from build123d import *

# Parameters (mm, degrees)
SKETCH1_R           = 1.45
BOSS_EXTRUDE1_DEPTH = 8
SKETCH2_R           = 4
SKETCH2_R_2         = 1.45
BOSS_EXTRUDE2_DEPTH = 2
SKETCH4_R           = 4
SKETCH4_R_2         = 2.75
BOSS_EXTRUDE3_DEPTH = 3
CUT_EXTRUDE1_DEPTH  = 3
CUT_EXTRUDE2_REACH  = 73.014
SKETCH6_R           = 1.5
CUT_EXTRUDE3_DEPTH  = 3
BOSS_EXTRUDE8_DEPTH = 5
BOSS_EXTRUDE9_START = -11
BOSS_EXTRUDE9_DEPTH = 4
CUT_EXTRUDE6_DEPTH  = 72.01408311
SKETCH6_7_R         = 1.5
CUT_EXTRUDE7_DEPTH  = 3


with BuildPart() as part:
    # Sketch1 → Boss-Extrude1 (new body)
    with BuildSketch(Plane(origin=(0, 0, 0), x_dir=(1, 0, 0), z_dir=(0, 1, 0))):
        with BuildLine():
            Line((-7.5, 36.5), (-43, 36.5))
            Line((-43, 36.5), (-43, 32.5))
            Line((-43, 32.5), (-17.5, 32.5))
            ThreePointArc((-17.5, 32.5), (-10.428932188, 29.571067812), (-7.5, 22.5))
            Line((-7.5, 22.5), (-7.5, 0))
            ThreePointArc((-7.5, 0), (0, -7.5), (7.5, 0))
            Line((7.5, 0), (7.5, 40))
            ThreePointArc((7.5, 40), (5.303300859, 45.303300859), (0, 47.5))
            Line((0, 47.5), (-19, 47.5))
            Line((-19, 47.5), (-19, 42.5))
            Line((-19, 42.5), (-7.5, 42.5))
            Line((-7.5, 42.5), (-7.5, 36.5))
        make_face()
        with Locations(Location((0, 0, 0), (0, 0, 270))):
            Circle(SKETCH1_R, mode=Mode.SUBTRACT)
        with BuildLine():
            ThreePointArc((-3.822328563, 25.208378945), (-4.975312132, 23.472395947), (-3.280610142, 22.259550844))
            ThreePointArc((-3.280610142, 22.259550844), (-0.06671842, 22.49990123), (3.148542183, 22.278615056))
            ThreePointArc((3.148542183, 22.278615056), (4.95957959, 23.370856111), (3.89359262, 25.197470135))
            ThreePointArc((3.89359262, 25.197470135), (0.03604708, 25.496495157), (-3.822328563, 25.208378945))
        make_face(mode=Mode.SUBTRACT)
    extrude(amount=BOSS_EXTRUDE1_DEPTH)

    # Sketch2 → Boss-Extrude2 (add)
    with BuildSketch(Plane(origin=(0, 8, 0), x_dir=(1, 0, 0), z_dir=(0, 1, 0))):
        with Locations(Location((0, 0, 0), (0, 0, 270))):
            Circle(SKETCH2_R)
        with Locations(Location((0, 0, 0), (0, 0, 270))):
            Circle(SKETCH2_R_2, mode=Mode.SUBTRACT)
    extrude(amount=BOSS_EXTRUDE2_DEPTH)

    # Sketch4 → Boss-Extrude3 (add)
    with BuildSketch(Plane(origin=(0, 10, 0), x_dir=(1, 0, 0), z_dir=(0, 1, 0))):
        with Locations(Location((0, 0, 0), (0, 0, 270))):
            Circle(SKETCH4_R)
        with Locations(Location((0, 0, 0), (0, 0, 270))):
            Circle(SKETCH4_R_2, mode=Mode.SUBTRACT)
    extrude(amount=BOSS_EXTRUDE3_DEPTH)

    # Sketch5 → Cut-Extrude1 (cut)
    with BuildSketch(Plane(origin=(0, 8, 0), x_dir=(1, 0, 0), z_dir=(0, 1, 0))):
        with BuildLine():
            ThreePointArc((-3.901041667, 26.464020366), (-6.220600225, 23.342378475), (-3.098958333, 21.022819917))
            ThreePointArc((-3.098958333, 21.022819917), (0, 21.25), (3.098958333, 21.022819917))
            ThreePointArc((3.098958333, 21.022819917), (6.220600225, 23.342378475), (3.901041667, 26.464020366))
            ThreePointArc((3.901041667, 26.464020366), (0, 26.75), (-3.901041667, 26.464020366))
        make_face()
    extrude(amount=-CUT_EXTRUDE1_DEPTH, mode=Mode.SUBTRACT)

    # Sketch6 → Cut-Extrude2 (cut, up to next)
    with BuildSketch(Plane(origin=(0, 0, -47.5), x_dir=(-1, 0, 0), z_dir=(0, 0, -1)), mode=Mode.PRIVATE) as cut_extrude2_sk1:
        with Locations((35, 4)):
            Circle(SKETCH6_R)
    cut_extrude2_tool1 = extrude(cut_extrude2_sk1.sketch, amount=-CUT_EXTRUDE2_REACH, mode=Mode.PRIVATE) & part.part
    # Sketch6 → Cut-Extrude2 (cut, up to next)
    with BuildSketch(Plane(origin=(0, 0, -47.5), x_dir=(-1, 0, 0), z_dir=(0, 0, -1)), mode=Mode.PRIVATE) as cut_extrude2_sk2:
        with BuildLine():
            ThreePointArc((13.205467269, 9.590021738), (12.125166536, 11.415658703), (10.299529571, 10.33535797))
            ThreePointArc((10.299529571, 10.33535797), (9.639691668, 6.665475813), (9.522099126, 2.938601373))
            ThreePointArc((9.522099126, 2.938601373), (11.083234391, 1.502336535), (12.519499229, 3.0634718))
            ThreePointArc((12.519499229, 3.0634718), (12.623257354, 6.351890424), (13.205467269, 9.590021738))
        make_face()
    cut_extrude2_tool2 = extrude(cut_extrude2_sk2.sketch, amount=-CUT_EXTRUDE2_REACH, mode=Mode.PRIVATE) & part.part
    add(cut_extrude2_tool1.solids().sort_by_distance((-35, 4, -47.5))[0], mode=Mode.SUBTRACT)
    add(cut_extrude2_tool2.solids().sort_by_distance((-11.259305, 6.495248, -47.5))[0], mode=Mode.SUBTRACT)

    # Sketch6<3> → Cut-Extrude3 (cut)
    with BuildSketch(Plane(origin=(0, 0, -47.5), x_dir=(-1, 0, 0), z_dir=(0, 0, -1))):
        with BuildLine():
            ThreePointArc((9.088722197, 10.645914733), (8.396539299, 6.796136392), (8.273182416, 2.886572028))
            ThreePointArc((8.273182416, 2.886572028), (11.135263735, 0.253419825), (13.768415938, 3.115501144))
            ThreePointArc((13.768415938, 3.115501144), (13.866409723, 6.221229844), (14.416274643, 9.279464975))
            ThreePointArc((14.416274643, 9.279464975), (12.435723299, 12.626466077), (9.088722197, 10.645914733))
        make_face()
        with BuildLine():
            ThreePointArc((10.299529571, 10.33535797), (9.639691668, 6.665475813), (9.522099126, 2.938601373))
            ThreePointArc((9.522099126, 2.938601373), (11.083234391, 1.502336535), (12.519499229, 3.0634718))
            ThreePointArc((12.519499229, 3.0634718), (12.623257354, 6.351890424), (13.205467269, 9.590021738))
            ThreePointArc((13.205467269, 9.590021738), (12.125166536, 11.415658703), (10.299529571, 10.33535797))
        make_face(mode=Mode.SUBTRACT)
    extrude(amount=-CUT_EXTRUDE3_DEPTH, mode=Mode.SUBTRACT)

    # Sketch8 → Boss-Extrude8 (add)
    with BuildSketch(Plane(origin=(0, 0, -47.5), x_dir=(-1, 0, 0), z_dir=(0, 0, -1))):
        with BuildLine():
            Line((19, 8), (19, 9.895699086))
            ThreePointArc((19, 9.895699086), (9.880775279, 12.931961804), (1.631235681, 8))
            Line((1.631235681, 8), (19, 8))
        make_face()
    extrude(amount=-BOSS_EXTRUDE8_DEPTH)

    # Sketch8<3> → Boss-Extrude9 (add)
    with BuildSketch(Plane(origin=(0, 0, -47.5), x_dir=(-1, 0, 0), z_dir=(0, 0, -1)).offset(BOSS_EXTRUDE9_START)):
        with BuildLine():
            Line((19, 8), (19, 9.895699086))
            ThreePointArc((19, 9.895699086), (9.880775279, 12.931961804), (1.631235681, 8))
            Line((1.631235681, 8), (19, 8))
        make_face()
    extrude(amount=-BOSS_EXTRUDE9_DEPTH)

    # Sketch6<6> → Cut-Extrude6 (cut, through all)
    with BuildSketch(Plane(origin=(0, 0, -47.5), x_dir=(-1, 0, 0), z_dir=(0, 0, -1))):
        with BuildLine():
            ThreePointArc((12.519499229, 3.0634718), (12.552838265, 5.541080797), (12.858410175, 8))
            Line((12.858410175, 8), (9.815679481, 8))
            ThreePointArc((9.815679481, 8), (9.542788681, 5.476615002), (9.522099126, 2.938601373))
            ThreePointArc((9.522099126, 2.938601373), (11.083234391, 1.502336535), (12.519499229, 3.0634718))
        make_face()
        with BuildLine():
            ThreePointArc((12.858410175, 8), (13.017557947, 8.798149788), (13.205467269, 9.590021738))
            ThreePointArc((13.205467269, 9.590021738), (12.125166536, 11.415658703), (10.299529571, 10.33535797))
            ThreePointArc((10.299529571, 10.33535797), (10.030287022, 9.17333875), (9.815679481, 8))
            Line((9.815679481, 8), (12.858410175, 8))
        make_face()
    extrude(amount=-CUT_EXTRUDE6_DEPTH, mode=Mode.SUBTRACT)

    # Sketch6<7> → Cut-Extrude7 (cut)
    # profile 1 of 2: a face of its own
    with BuildSketch(Plane(origin=(0, 0, -47.5), x_dir=(-1, 0, 0), z_dir=(0, 0, -1))):
        with Locations((35, 4)):
            Circle(SKETCH6_7_R)
    # profile 2 of 2: a face of its own
    with BuildSketch(Plane(origin=(0, 0, -47.5), x_dir=(-1, 0, 0), z_dir=(0, 0, -1))):
        with BuildLine():
            ThreePointArc((14.416274643, 9.279464975), (13.866409723, 6.221229844), (13.768415938, 3.115501144))
            ThreePointArc((13.768415938, 3.115501144), (11.135263735, 0.253419825), (8.273182416, 2.886572028))
            ThreePointArc((8.273182416, 2.886572028), (8.396539299, 6.796136392), (9.088722197, 10.645914733))
            ThreePointArc((9.088722197, 10.645914733), (12.435723299, 12.626466077), (14.416274643, 9.279464975))
        make_face()
        with BuildLine():
            ThreePointArc((13.205467269, 9.590021738), (12.125166536, 11.415658703), (10.299529571, 10.33535797))
            ThreePointArc((10.299529571, 10.33535797), (9.639691668, 6.665475813), (9.522099126, 2.938601373))
            ThreePointArc((9.522099126, 2.938601373), (11.083234391, 1.502336535), (12.519499229, 3.0634718))
            ThreePointArc((12.519499229, 3.0634718), (12.623257354, 6.351890424), (13.205467269, 9.590021738))
        make_face(mode=Mode.SUBTRACT)
    extrude(amount=-CUT_EXTRUDE7_DEPTH, mode=Mode.SUBTRACT)


solid = part.part
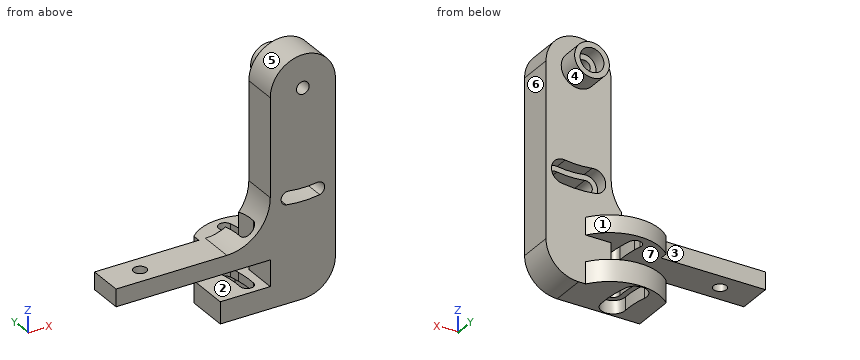
For this review, take the finished solid that the model builds, in its own axes (mm). Face numbers are marked on the shaded views. A direction names the side the tool comes from. Coordinates: 2 decimals unless noted, no trailing zeros. Order: outer loops, then holes, each group sorted by start corner. A loop starts at its lowest first (then second) coordinate and runs counter-clockwise, first axis right, second up. Notation, with made-up numbers: (37, -38.5) - (74, -38.5) arc R30 ccw to (74, -11.5) - close; hole circle Ø9 at (46.5, 62). An arc over 180 degrees is marked (long way). Answer as CSV lines item,"result". Start each with the question number.
1) To check wall thickness, follow line 1 along Y through (x, z) = (-35, -35); line 2 along X through (y, z) = (12.4, 0); line 3 along Z through (x, y) = (-17.5, 9.25). State the ranges of each line that lie inside material, in increasing order. Write a range as [from, to].
2) Machinability: for the marked faces 1, 2, 3 and 4, which of the approach directions +Z, -Z, +X, -X, +Y, -Y give a long, thin tool a straight path to every point of the face, cutting with its end or side? Answer none if there is none.
3) Add section B-B (y = 6.5). Count the separate pieces of the cut face and the enclosed holes in it, then the cut area to 3 significant figures.
4) Insertion check: P1, Ø6.5, axis at x = 2.5, z = -24, coming from the +Y side; P2, Ø4, axis at y = 6.5, z = -46, coming from the -X side; P3, Ø2, axis at y = 8.5, z = -35, coming from the -X side; P4, Ø3, axis at x = -23.5, y = 5, coming from the -Z side. Each pin has a flat end and moves straight along its axis. Give the tip position at first contact, or say it passes through.
5) Add section A-A (x = -35). State the section outline as (y, z) points.
6) Draft analysis for pull direction Z (two halves, no side actions). For the marked faces 5, 6 and 7, state which applies: +Z half, -Z half, draft (parallel to the pull), parting line (faces both ways), or undercut.
Result:
1,line 1,"[0, 2.5], [5.5, 8]"
1,line 2,"[-4, -2.75], [2.75, 4]"
1,line 3,"[-47.5, -42.5], [-36.5, -32.5]"
2,face 1,"-Z, +Y"
2,face 2,"-X, +Y"
2,face 3,"+Z, -Z, -X, +Y"
2,face 4,"+Y"
3,separate pieces,"3"
3,enclosed holes,"2"
3,area,"899 mm^2"
4,P1,"y = 8"
4,P2,"x = -19"
4,P3,"x = -43"
4,P4,"z = -36.5"
5,outline,"(0, -36.5) - (2.5, -36.5) - (2.5, -32.5) - (0, -32.5) - close; (5.5, -36.5) - (8, -36.5) - (8, -32.5) - (5.5, -32.5) - close"
6,face 5,"+Z half"
6,face 6,"draft"
6,face 7,"undercut"
